The drawing under review shows one solid part. Ordinate dimensions are in mm from its lowest x, y, z. A direction names the side the tool comes from. Round coordinates to 2 decimals unless told otherwise and drop trailing zeros. Order: outer loops, then holes, each group sorted by start corner. A loop starts at its lowest first (then second) coordinate and runs counter-clockwise, first axis right, second up. Notation, with made-up numbers: M 77.25,71 L 125.25,71 A19 cw 125.25,108 Z; hole C 36,89.25 d3. An arc over 180 degrees is marked long. Answer as a JSON object with one key per item and string values.
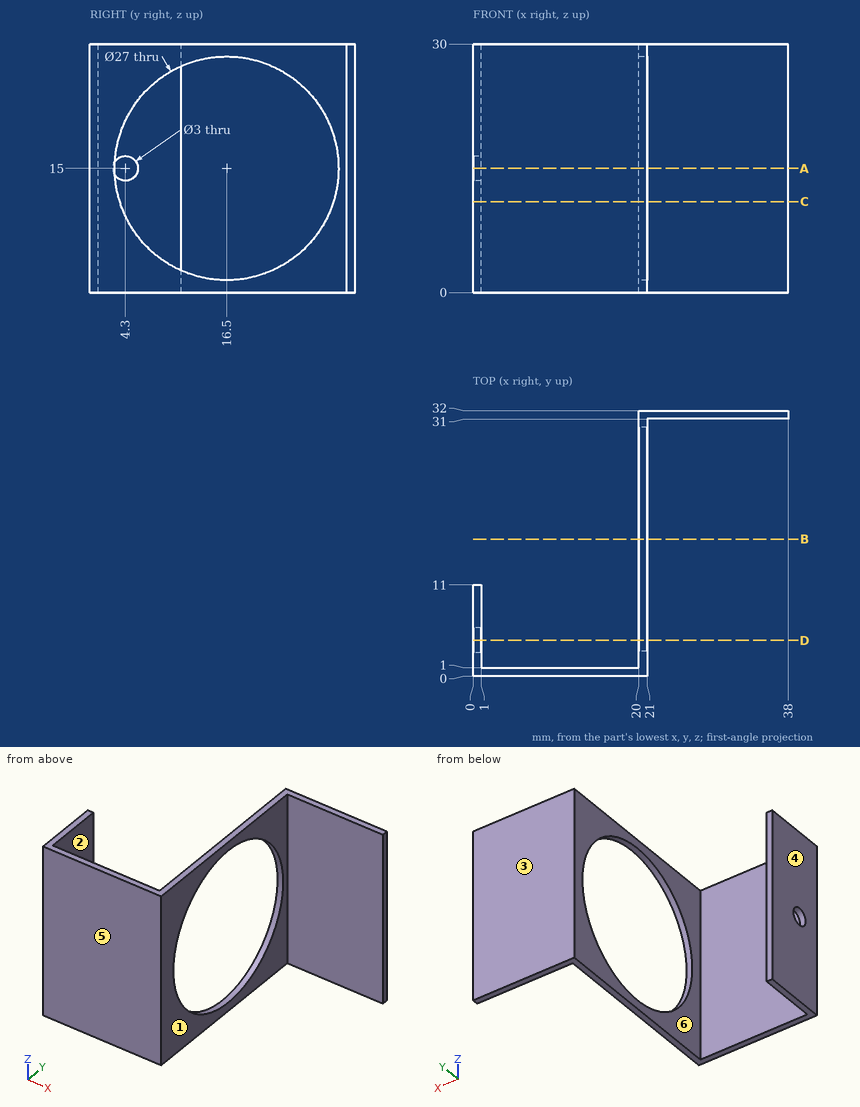
1) Mouldability with a two-part tool opening along X and no side actions: class the marked faces 4, 5 and 6 as +X half, -X half, draft (parallel to the pull), parting line (faces both ways), or undercut.
Geometry check:
{"face 4": "-X half", "face 5": "draft", "face 6": "undercut"}
2) Add section C-C on z = 11. State the section outline as (x, y) points, and give its area (3 significant figures).
Geometry check:
{"outline": "M 0,0 L 21,0 L 21,3.61 L 20,3.61 L 20,1 L 1,1 L 1,11 L 0,11 Z; M 20,29.39 L 21,29.39 L 21,31 L 38,31 L 38,32 L 20,32 Z", "area": "53.2 mm²"}
3) Add section D-D on y = 4.3. State the section outline as (x, z) points.
Geometry check:
{"outline": "M 0,0 L 1,0 L 1,13.5 L 0,13.5 Z; M 0,16.5 L 1,16.5 L 1,30 L 0,30 Z; M 20,0 L 21,0 L 21,9.22 L 20,9.22 Z; M 20,20.78 L 21,20.78 L 21,30 L 20,30 Z"}
4) Machinability: for the marked faces 1, 2 and 3, which of the approach directions +Z, -Z, +X, -X, +Y, -Y give a long, thin tool a straight path to every point of the face, cutting with its end or side? Answer none if there is none.
Geometry check:
{"face 1": "+Z, -Z, +X, -Y", "face 2": "+Z, -Z, +Y", "face 3": "+Z, -Z, +X, -X, +Y"}
5) Add section B-B on y = 16.5. State the section outline as (x, z) points.
Geometry check:
{"outline": "M 20,0 L 21,0 L 21,1.5 L 20,1.5 Z; M 20,28.5 L 21,28.5 L 21,30 L 20,30 Z"}
6) For L1, parallel to X at y = 6, z = 3.75; L2, parallel to Y at x = 20.5, z = 15; L3, parallel to Y at x = 0.6, z = 15, list the stretches that pass through material, from the lowest coordinate up.
Geometry check:
{"L1": "x = 0 to 1, 20 to 21", "L2": "y = 0 to 3, 30 to 32", "L3": "y = 0 to 2.8, 5.8 to 11"}
7) Add section A-A on z = 15. State the section outline as (x, y) points, and give its area (3 significant figures).
Geometry check:
{"outline": "M 0,0 L 21,0 L 21,3 L 20,3 L 20,1 L 1,1 L 1,2.8 L 0,2.8 Z; M 0,5.8 L 1,5.8 L 1,11 L 0,11 Z; M 20,30 L 21,30 L 21,31 L 38,31 L 38,32 L 20,32 Z", "area": "49.0 mm²"}
8) Insertion check: P1, Ø5.5, axis at x = 9, z = 10, coming from the +Y side; P2, Ø11, axis at y = 7, z = 20.5, coming from the +X side; P3, Ø0.8, axis at x = 0.5, z = 15.5, coming from the +Y side. Each pin has a flat end and moves straight along its axis. Give the tip position at first contact, or say it passes through.
Geometry check:
{"P1": "stops at y = 1", "P2": "stops at x = 21", "P3": "stops at y = 11"}
